from build123d import *

# Parameters (mm, degrees)
ESQUISSE1_W             = 20.2
ESQUISSE1_H             = 8.4
BOSS_EXTRU_1_DEPTH      = 12.2
ENL_V_MAT_EXTRU_1_DEPTH = 8.5
ESQUISSE3_W             = 4.3
ESQUISSE3_H             = 0.5
ENL_V_MAT_EXTRU_2_DEPTH = 21.2
ESQUISSE4_R             = 0.6
BOSS_EXTRU_2_DEPTH      = 4
BOSS_EXTRU_2_DEPTH_BACK = 11.5
CHANFREIN1_SIZE         = 0.2
CHANFREIN1_SIZE2        = 0.746410162
CHANFREIN1_PART_2_SIZE  = 0.2
CHANFREIN1_PART_2_SIZE2 = 0.746410162
CHANFREIN1_PART_3_SIZE  = 0.2
CHANFREIN1_PART_3_SIZE2 = 0.746410162
CHANFREIN1_PART_4_SIZE  = 0.2
CHANFREIN1_PART_4_SIZE2 = 0.746410162
CHANFREIN2_SIZE         = 0.2
ESQUISSE5_R             = 1.1
BOSS_EXTRU_3_DEPTH      = 0.6


with BuildPart() as part:
    # Esquisse1 → Boss.-Extru.1 (new body)
    with BuildSketch(Plane.XY):
        with Locations((10.1, 4.2)):
            Rectangle(ESQUISSE1_W, ESQUISSE1_H)
    extrude(amount=BOSS_EXTRU_1_DEPTH)

    # Esquisse2 → Enlèv. mat.-Extru.1 (cut)
    with BuildSketch(Plane.XY.offset(12.2)):
        with BuildLine():
            Line((0, 1.4), (0, 6.9))
            Line((0, 6.9), (20.2, 6.9))
            Line((20.2, 6.9), (20.2, 1.4))
            Line((20.2, 1.4), (19.52, 1.4))
            ThreePointArc((19.52, 1.4), (17.72, 0.8), (15.92, 1.4))
            Line((15.92, 1.4), (14.44, 1.4))
            ThreePointArc((14.44, 1.4), (12.64, 0.8), (10.84, 1.4))
            Line((10.84, 1.4), (9.36, 1.4))
            ThreePointArc((9.36, 1.4), (7.56, 0.8), (5.76, 1.4))
            Line((5.76, 1.4), (4.28, 1.4))
            ThreePointArc((4.28, 1.4), (2.48, 0.8), (0.68, 1.4))
            Line((0.68, 1.4), (0, 1.4))
        make_face()
    extrude(amount=-ENL_V_MAT_EXTRU_1_DEPTH, mode=Mode.SUBTRACT)

    # Esquisse3 → Enlèv. mat.-Extru.2 (cut, through all)
    with BuildSketch(Plane.ZY):
        with Locations((6.85, 8.15)):
            Rectangle(ESQUISSE3_W, ESQUISSE3_H)
        Polygon((12.2, 8.4), (9.2, 8.4), (12.2, 8.05), align=None)
        Polygon((12.2, 7.25), (12.2, 6.9), (9.2, 6.9), align=None)
    extrude(amount=-ENL_V_MAT_EXTRU_2_DEPTH, mode=Mode.SUBTRACT)

    # Esquisse4 → Boss.-Extru.2 (add, two sides)
    with BuildSketch(Plane(origin=(0, 0, 0), x_dir=(-1, 0, 0), z_dir=(0, 0, -1))) as boss_extru_2_sk:
        with Locations((-17.72, 3.75)):
            Circle(ESQUISSE4_R)
        with Locations((-12.64, 3.75)):
            Circle(ESQUISSE4_R)
        with Locations((-2.48, 3.75)):
            Circle(ESQUISSE4_R)
        with Locations((-7.56, 3.75)):
            Circle(ESQUISSE4_R)
    extrude(amount=BOSS_EXTRU_2_DEPTH)
    extrude(boss_extru_2_sk.sketch, amount=-BOSS_EXTRU_2_DEPTH_BACK)

    # Chanfrein1
    chanfrein1_edges = [part.edges().sort_by_distance(p)[0] for p in [
        (8.16, 3.75, 11.5),
    ]]
    chanfrein1_side = [part.faces().sort_by_distance(p)[0] for p in [
        (7.56, 3.75, 11.5),
    ]]
    chamfer(chanfrein1_edges, length=CHANFREIN1_SIZE, length2=CHANFREIN1_SIZE2, reference=chanfrein1_side[0])

    # Chanfrein1 part 2
    chanfrein1_part_2_edges = [part.edges().sort_by_distance(p)[0] for p in [
        (18.32, 3.75, 11.5),
    ]]
    chanfrein1_part_2_side = [part.faces().sort_by_distance(p)[0] for p in [
        (17.72, 3.75, 11.5),
    ]]
    chamfer(chanfrein1_part_2_edges, length=CHANFREIN1_PART_2_SIZE, length2=CHANFREIN1_PART_2_SIZE2, reference=chanfrein1_part_2_side[0])

    # Chanfrein1 part 3
    chanfrein1_part_3_edges = [part.edges().sort_by_distance(p)[0] for p in [
        (13.24, 3.75, 11.5),
    ]]
    chanfrein1_part_3_side = [part.faces().sort_by_distance(p)[0] for p in [
        (12.64, 3.75, 11.5),
    ]]
    chamfer(chanfrein1_part_3_edges, length=CHANFREIN1_PART_3_SIZE, length2=CHANFREIN1_PART_3_SIZE2, reference=chanfrein1_part_3_side[0])

    # Chanfrein1 part 4
    chanfrein1_part_4_edges = [part.edges().sort_by_distance(p)[0] for p in [
        (3.08, 3.75, 11.5),
    ]]
    chanfrein1_part_4_side = [part.faces().sort_by_distance(p)[0] for p in [
        (2.48, 3.75, 11.5),
    ]]
    chamfer(chanfrein1_part_4_edges, length=CHANFREIN1_PART_4_SIZE, length2=CHANFREIN1_PART_4_SIZE2, reference=chanfrein1_part_4_side[0])

    # Chanfrein2
    chanfrein2_edges = [part.edges().sort_by_distance(p)[0] for p in [
        (8.16, 3.75, -4),
        (18.32, 3.75, -4),
        (13.24, 3.75, -4),
        (3.08, 3.75, -4),
    ]]
    chamfer(chanfrein2_edges, length=CHANFREIN2_SIZE)

    # Esquisse5 → Boss.-Extru.3 (add)
    with BuildSketch(Plane.XY.offset(3.7)):
        with Locations((12.64, 3.75)):
            Circle(ESQUISSE5_R)
        with Locations((17.72, 3.75)):
            Circle(ESQUISSE5_R)
        with Locations((7.56, 3.75)):
            Circle(ESQUISSE5_R)
        with Locations((2.48, 3.75)):
            Circle(ESQUISSE5_R)
    extrude(amount=BOSS_EXTRU_3_DEPTH)


solid = part.part
Design review of the part built by this model. Coordinates are the model's own, in mm. A direction names the side the tool comes from. Coordinates: 2 decimals unless noted, no trailing zeros. Order: outer loops, then holes, each group sorted by start corner. A loop starts at its lowest first (then second) coordinate and runs counter-clockwise, first axis right, second up. Notation, with made-up numbers: (5, -23) -> (47, -23) arc R19 ccw to (47, 10) -> close; hole circle Ø2 at (66, 10). An arc over 180 degrees is marked (long way). Use one line per item in the form item = value. Start each with the question number.
(1) Insertion check: pin 1 (1.5 mm diameter, centred on y = 4, z = 5, fed in from +X); pin 2 (1.1 mm diameter, centred on x = 2, y = 3.5, fed in from +Z); pin 3 (2 mm diameter, centred on x = 11, z = 7.5, fed in from +Y). Each pin has a flat end and moves straight along its axis. Give the tip position at first contact, or say it passes through.
(2) Add section A-A on z = 6.25. State the section outline as (x, y) points.
(3) Add section D-D on y = 6.25. State the section outline as (x, z) points, plus the area to 3 significant figures.
(4) Add section C-C on z = -3. State the section outline as (x, y) points, plus the area to 3 significant figures.
(5) For probe 1 along Y at (x, z) = (9.75, 7.25); probe 2 along Z at (x, y) = (16.25, 3); probe 3 along Z at (x, y) = (13.75, 0.5), list the stretches that pass through material, from the lowest coordinate up.
(6) The part is to be moulded in two halves that separate along Y. For faces 5 (the flat face through (10, 4, 3.7)), 6 (the flat face through (20.2, 4, 3)), 7 (the flat face through (10, 7.9, 7)), say which applies: +Y half, -Y half, draft (parallel to the pull), parting line (faces both ways), or undercut.
(7) For faces 1 (the flat face through (10, 7.7, 12.2)), 2 (the cylindrical face through (6.988, 3.93, -1.873)), 3 (the flat face through (7.6, 3.8, 11.5)), 4 (the cylindrical face through (17.7, 0.8, 8)), list the 3-axis set-ups (+Z, -Z, +X, -X, +Y, -Y) from which the entire face can be reached by the end or side of a thin tool; tool diameter is ignored.
Answer block:
q1.pin_1 = 18.82
q1.pin_2 = 11.5
q1.pin_3 = 7.9
q2.outline = (0, 0) -> (20.2, 0) -> (20.2, 1.4) -> (19.52, 1.4) arc R3 cw to (15.92, 1.4) -> (14.44, 1.4) arc R3 cw to (10.84, 1.4) -> (9.36, 1.4) arc R3 cw to (5.76, 1.4) -> (4.28, 1.4) arc R3 cw to (0.68, 1.4) -> (0, 1.4) -> close; (0, 6.9) -> (20.2, 6.9) -> (20.2, 7.9) -> (0, 7.9) -> close; circle Ø1.2 at (2.48, 3.75); circle Ø1.2 at (7.56, 3.75); circle Ø1.2 at (12.64, 3.75); circle Ø1.2 at (17.72, 3.75)
q3.outline = (0, 0) -> (20.2, 0) -> (20.2, 3.7) -> (0, 3.7) -> close
q3.area = 74.7 mm²
q4.outline = circle Ø1.2 at (2.48, 3.75); circle Ø1.2 at (7.56, 3.75); circle Ø1.2 at (12.64, 3.75); circle Ø1.2 at (17.72, 3.75)
q4.area = 4.52 mm²
q5.probe_1 = 0 to 1.4, 6.9 to 7.9
q5.probe_2 = 0 to 3.7
q5.probe_3 = 0 to 12.2
q6.face_5 = undercut
q6.face_6 = draft
q6.face_7 = +Y half
q7.face_1 = +Z, +X, -X, +Y, -Y
q7.face_2 = -Z
q7.face_3 = +Z, +X, -X
q7.face_4 = +Z
